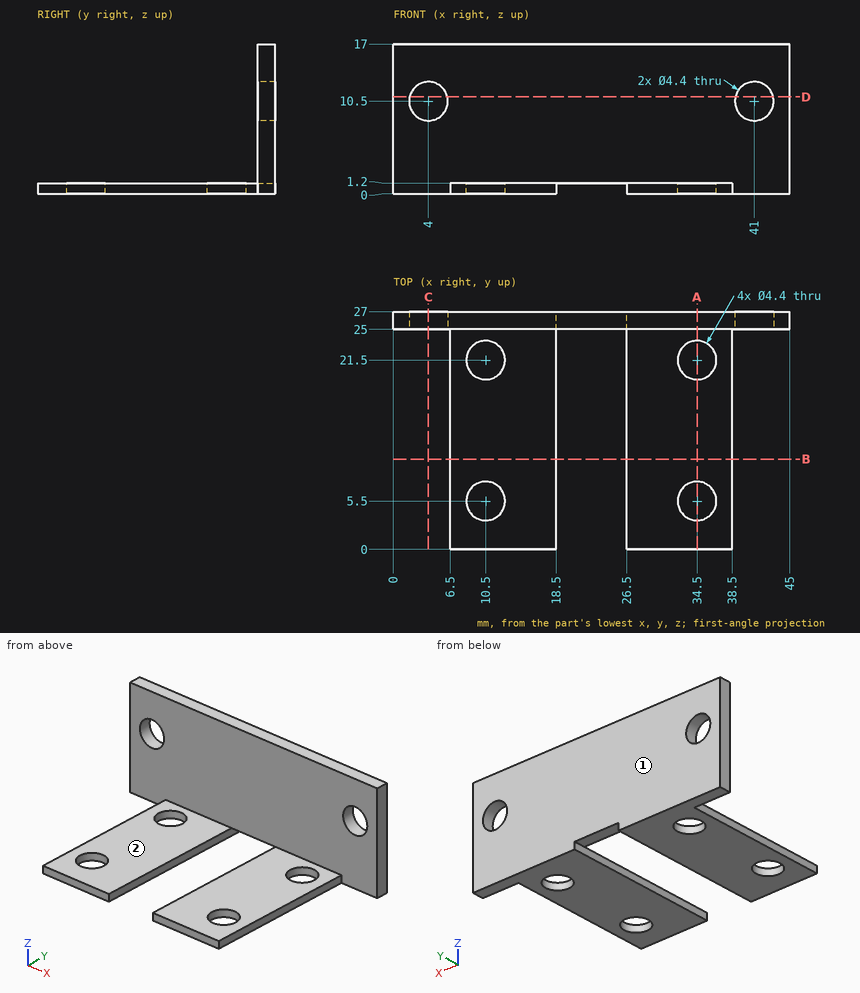
Answer from the drawing. Dimensions are ordinates in mm from the lowest x, y and z of the part. A direction names the side the tool comes from. Coordinates: 2 decimals unless noted, no trailing zeros. Write each loop counter-clockwise with the first axis right and the second up, starting at its lowest first coordinate (ties: lowest second). Pieces come first, ordered by that corner, then holes. Notation, with made-up numbers: M 6,83.5 L 21,83.5 A27 ccw 21,114.5 Z; hole C 62,19.25 d3. An arc over 180 degrees is marked long. Use one line per item in the form item = value. Start each with the question number.
1. The part is cut by section C-C (x = 4). Give the vertices of the cut face in (y, z).
2. Each of these flat-tipped pins is pushed along its axis until it touches: P1, Ø2.5, axis at x = 10.5, y = 5.5, coming from the -Z side; P2, Ø1, axis at y = 7.5, z = 0.5, coming from the -X side; P3, Ø1.3, axis at y = 11, z = 0.5, coming from the +X side; P4, Ø1.6, axis at x = 22.5, y = 26.5, coming from the -Z side. Where does it stop, or does it pass through?
3. The part is cut by section D-D (z = 11). Give the vertices of the cut face in (x, y).
4. A tool of negligible diameter and unlimited length cuts with its end or side. For the marked faces 1 and 2, from which of +Z, -Z, +X, -X, +Y, -Y can it reach the whole face along a straight path? Write none if from no direction.
5. Straight lines are drawn through the part: probe 1 along X at (y, z) = (21.5, 0.95); probe 2 along Y at (x, z) = (10.5, 0.85); probe 3 along Z at (x, y) = (41, 25.95). For each, find the intervals that lie inside material, in ascending order. Write a range as from..to.
6. The part is cut by section B-B (y = 10.25). Give the vertices of the cut face in (x, z).
7. The part is cut by section A-A (x = 34.5). Give the vertices of the cut face in (y, z), plus the area to 3 significant figures.
Evaluation:
q1.outline = M 25,0 L 27,0 L 27,8.3 L 25,8.3 Z; M 25,12.7 L 27,12.7 L 27,17 L 25,17 Z
q2.P1 = through
q2.P2 = 6.5
q2.P3 = 38.5
q2.P4 = 1.2
q3.outline = M 0,25 L 1.86,25 L 1.86,27 L 0,27 Z; M 6.14,25 L 38.86,25 L 38.86,27 L 6.14,27 Z; M 43.14,25 L 45,25 L 45,27 L 43.14,27 Z
q4.face_1 = +Z, -Z, +X, -X, +Y
q4.face_2 = +Z, +X, -X, -Y
q5.probe_1 = 6.5..8.3, 12.7..18.5, 26.5..32.3, 36.7..38.5
q5.probe_2 = 0..3.3, 7.7..19.3, 23.7..27
q5.probe_3 = 0..8.3, 12.7..17
q6.outline = M 6.5,0 L 18.5,0 L 18.5,1.2 L 6.5,1.2 Z; M 26.5,0 L 38.5,0 L 38.5,1.2 L 26.5,1.2 Z
q7.outline = M 0,0 L 3.3,0 L 3.3,1.2 L 0,1.2 Z; M 7.7,0 L 19.3,0 L 19.3,1.2 L 7.7,1.2 Z; M 23.7,0 L 27,0 L 27,17 L 25,17 L 25,1.2 L 23.7,1.2 Z
q7.area = 53.4 mm^2
